Input: dimensioned drawing with shaded views. Units: mm. Origin: part minimum x, y, z. A direction names the side the tool comes from. Round coordinates to 2 decimals unless told otherwise and drop trailing zeros. Loops run counter-clockwise (first coordinate to the right, second up) from the corner with the lowest first, then second, coordinate; pieces in that order, holes last. Notation, with made-up numbers: M 25,10 L 70,10 A31 cw 70,37 Z; hole C -14.5,16 d10. An arc over 180 degrees is marked long. Put each result on its own line as item: value. Start each with the question number.
1) Line query: probe 1 along X at (y, z) = (6.5, 7); probe 2 along Z at (x, y) = (1.1, 5.5); probe 3 along Y at (x, z) = (3.3, 4) (1 decimal). Output: solid intervals per line, ascending.
2) Section D-D on x = 3.2. Output: boundary loops of the cut face in (y, z).
3) Section B-B on y = 4.25. Output: boundary loops of the cut face in (x, z).
4) Draft query along Z for the marked faces 1, 2, 3 and 4. Return one class per face: +Z half, -Z half, draft (parallel to the pull), parting line (faces both ways), or undercut.
5) Pin query (flat end, axial travel): pin 1 (2 mm diameter, centred on x = 2.5, y = 6, fed in from -Z); pin 2 (0.5 mm diameter, centred on x = 0.5, z = 4, fed in from +Y); pin 3 (3 mm diameter, centred on x = 4, z = 4, fed in from -Y). Return the tip coordinate at first contact, or that it passes through.
6) Reachability of the marked faces 5 and 6 from +Z, -Z, +X, -X, +Y, -Y: full face, straight path, thin tool, end or side. Return the list, or none.
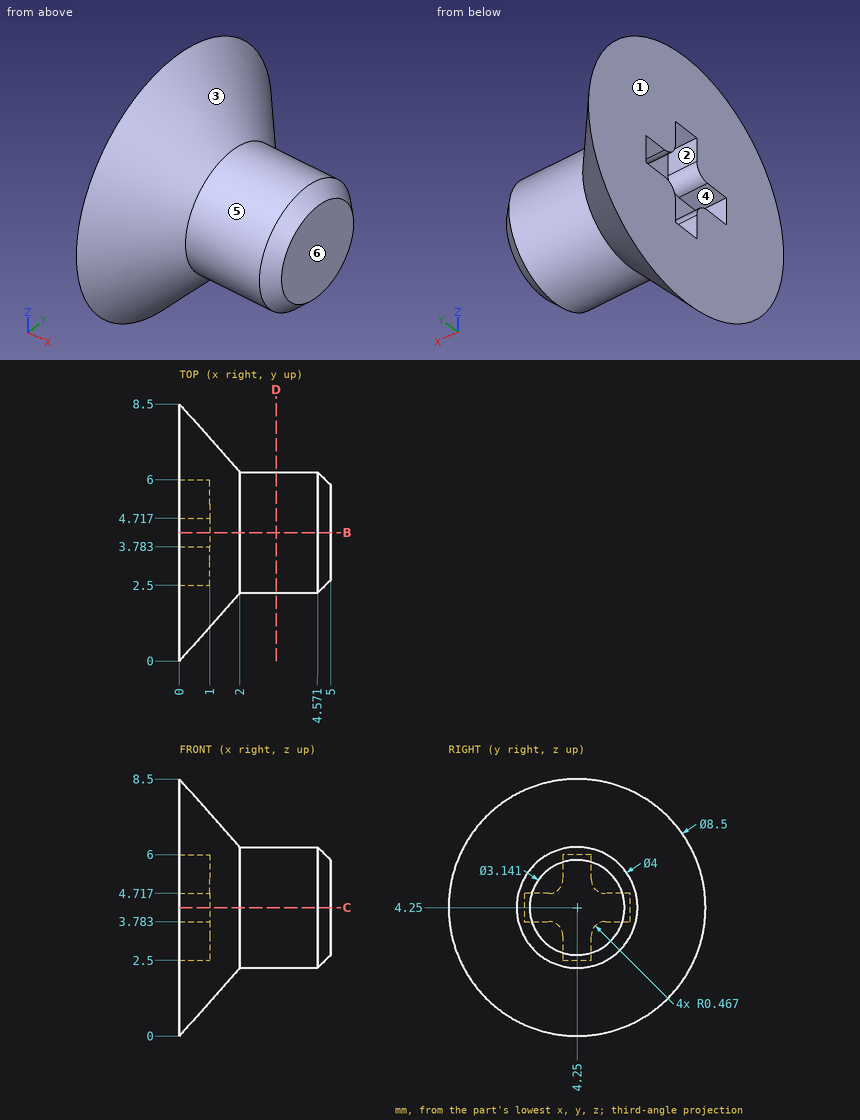
Geometry results:
1. probe 1: x = 0 to 0.62
1. probe 2: z = 1.51 to 6.99
1. probe 3: y = 2.3 to 6.2
2. outline: C 4.25,4.25 d4
3. outline: M 0,0 L 2,2.25 L 4.57,2.25 L 5,2.68 L 5,5.82 L 4.57,6.25 L 2,6.25 L 0,8.5 L 0,6 L 1,6 L 1,2.5 L 0,2.5 Z
4. face 1: draft
4. face 2: undercut
4. face 3: parting line
4. face 4: undercut
5. pin 1: stops at z = 2.18
5. pin 2: stops at y = 8.21
5. pin 3: stops at y = 2.25
6. face 5: +X
6. face 6: +Z, -Z, +X, +Y, -Y
